Geometry check sheet. Reference: drawing and pictorial views, mm from the part's lowest x, y, z. A direction names the side the tool comes from. Coordinates: 2 decimals unless noted, no trailing zeros. Loops run counter-clockwise (first coordinate to the right, second up) from the corner with the lowest first, then second, coordinate; pieces in that order, holes last.
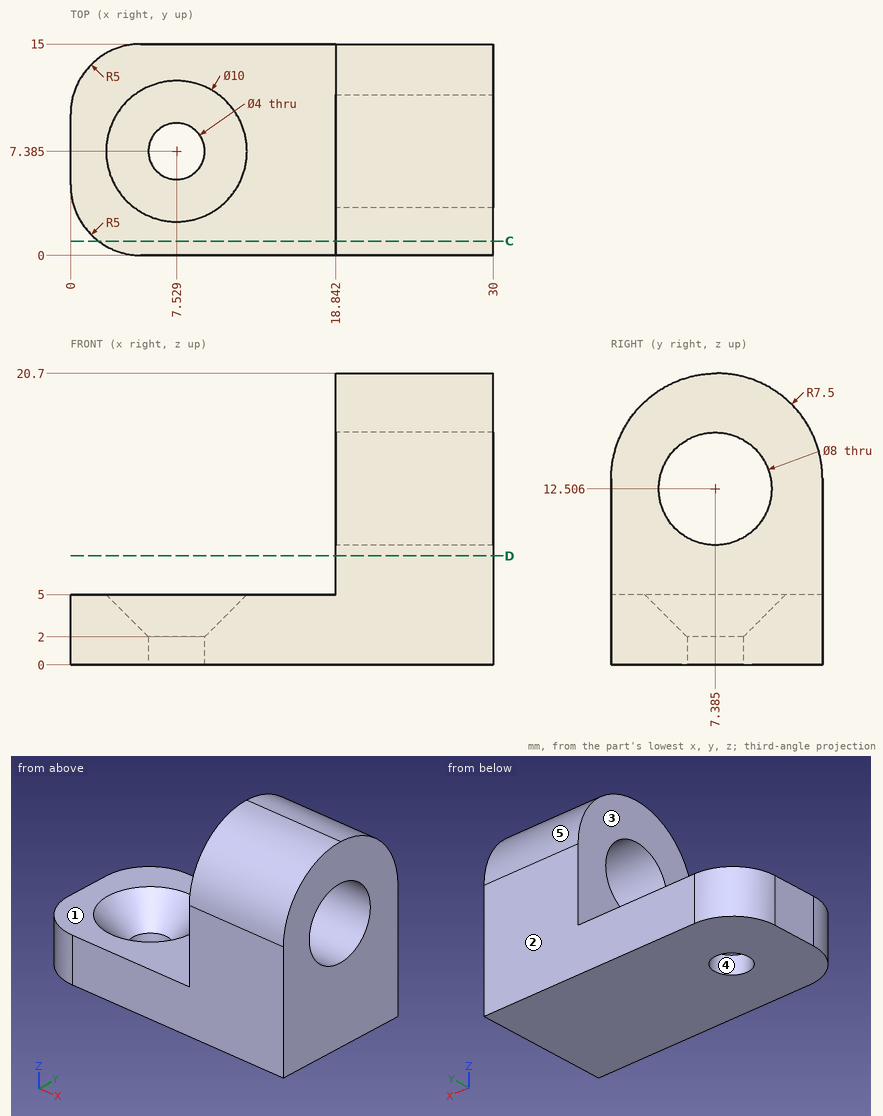
1) Depth check by flat-ended pin: pin 1 (5 mm diameter, centred on x = 3, y = 4, fed in from -Z); pin 2 (4 mm diameter, centred on x = 13, z = 8, fed in from -Y); pin 3 (2 mm diameter, centred on x = 24, y = 5.5, fed in from +Z). Enter the tip coordinate at first touch or a pass-through.
Data:
pin 1: stops at z = 0
pin 2: passes through
pin 3: stops at z = 20.63
2) Material ranges on probe 1 along Y at (x, z) = (24, 12.5) (1 decimal); probe 2 along X at (y, z) = (1, 11.5); probe 3 along Z at (x, y) = (25.5, 10) (1 decimal), recorded low to high.
Data:
probe 1: y = 0 to 3.4, 11.4 to 15
probe 2: x = 18.84 to 30
probe 3: z = 0 to 9.5, 15.5 to 20.3
3) Section check C-C on y = 1. Record the cut outline in (x, z), and give its area (3 significant figures).
Data:
outline: (2, 0) - (30, 0) - (30, 16.94) - (18.84, 16.94) - (18.84, 5) - (2, 5) - close
area: 273 mm2
4) Section check D-D on z = 7.75. Record the cut outline in (x, y), and give its area (3 significant figures).
Data:
outline: (18.84, 0) - (30, 0) - (30, 15) - (18.84, 15) - close
area: 167 mm2
5) Access from +Z, -Z, +X, -X, +Y, -Y to the whole of each face (thin tool, end or side, straight path). Record for the marked faces 1 and 2.
Data:
face 1: +Z, -X, +Y, -Y
face 2: +Z, -Z, +X, -X, +Y
6) Mould release check, pull along X, two halves, no side actions. Record for the marked faces 3, 4 and 5: +X half, -X half, draft (parallel to the pull), parting line (faces both ways), or undercut.
Data:
face 3: -X half
face 4: undercut
face 5: draft
